The model under review builds one solid part; all positions refer to its coordinate system, in mm. Coordinates: 2 decimals unless noted, no trailing zeros. Order: outer loops, then holes, each group sorted by start corner. A loop starts at its lowest first (then second) coordinate and runs counter-clockwise, first axis right, second up. Notation, with made-up numbers: M 48.25,-39.75 L 99.25,-39.75 A29 ccw 99.25,-3.75 Z; hole C 67.25,22 d1. An arc over 180 degrees is marked long. Write each question's results on one line, items separated by ' | '.
from build123d import *

# Parameters (mm, degrees)
SKETCH1_W                                    = 40
SKETCH1_H                                    = 10
BOSS_EXTRUDE1_DEPTH                          = 3
CSK_FOR_M3_COUNTERSUNK_FLAT_HEAD_SCR_2_COUNT = 2
CSK_FOR_M3_COUNTERSUNK_FLAT_HEAD_SCR_2_PITCH = 28


with BuildPart() as part:
    # Sketch1 → Boss-Extrude1 (new body)
    with BuildSketch(Plane(origin=(0, 0, 0), x_dir=(1, 0, 0), z_dir=(0, 1, 0))):
        Rectangle(SKETCH1_W, SKETCH1_H)
    extrude(amount=BOSS_EXTRUDE1_DEPTH)

    # Sketch3 → CSK for M3 Countersunk Flat Head Screw1 (revolve, cut)
    with BuildSketch(Plane(origin=(-14, 3, 0), x_dir=(0, 0, 1), z_dir=(1, 0, 0))):
        Polygon((0, 0), (0, 3), (1.7, 3), (1.7, 1.45), (3.15, 0), align=None)
    csk_for_m3_countersunk_flat_head_screw1 = revolve(axis=Axis((-14, 9.35, 0), (0, -1, 0)), mode=Mode.SUBTRACT)

    # CSK for M3 Countersunk Flat Head Scr 2: CSK for M3 Countersunk Flat Head Screw1 ×2
    with Locations(*[(i * CSK_FOR_M3_COUNTERSUNK_FLAT_HEAD_SCR_2_PITCH, 0, 0) for i in range(1, CSK_FOR_M3_COUNTERSUNK_FLAT_HEAD_SCR_2_COUNT)]):
        add(csk_for_m3_countersunk_flat_head_screw1, mode=Mode.SUBTRACT)


solid = part.part
1) Take a section at B-B on z = 0. State the section outline as (x, y) points, plus the area to 3 significant figures.
Solutions:
outline: M -20,0 L -15.7,0 L -15.7,1.55 L -17.15,3 L -20,3 Z; M -12.3,0 L 12.3,0 L 12.3,1.55 L 10.85,3 L -10.85,3 L -12.3,1.55 Z; M 15.7,0 L 20,0 L 20,3 L 17.15,3 L 15.7,1.55 Z | area: 95.4 mm2
2) To check wall thickness, follow line 1 along X through (y, z) = (1.05, 0); line 2 along Z through (x, y) = (-14, 0.55); line 3 along X through (y, z) = (1.2, -1). State the ranges of each line that lie inside material, in increasing order.
Solutions:
line 1: -20 to -15.7, -12.3 to 12.3, 15.7 to 20 | line 2: -5 to -1.7, 1.7 to 5 | line 3: -20 to -15.37, -12.63 to 12.63, 15.37 to 20
3) Take a section at C-C on y = 1.15. State the section outline as (x, z) points.
Solutions:
outline: M -20,-5 L 20,-5 L 20,5 L -20,5 Z; hole C -14,0 d3.4; hole C 14,0 d3.4
4) For pin 1 (4 mm diameter, centred on x = 10, z = 3, fed in from -Y); pin 2 (2.5 mm diameter, centred on x = -14, z = 0, fed in from +Y), all flat-tipped, find the tip position at first contact; note any pin that passes through.
Solutions:
pin 1: y = 0 | pin 2: through
5) The part is to be moulded in two halves that separate along X. For faces 1 (the flat face through (-20, 1, 0)), 2 (the cylindrical face through (12.314, 0.786, -0.221)), 3 (the flat face through (0, 0, 0)), 4 (the flat face through (20, 1, 0)), say which applies: pulls with the +X half, pulls with the -X half, needs draft (parallel to the pull), parting line crosses it, or undercut.
Solutions:
face 1: pulls with the -X half | face 2: undercut | face 3: needs draft | face 4: pulls with the +X half
6) Take a section at A-A on x = -14. State the section outline as (y, z) points.
Solutions:
outline: M 0,-5 L 3,-5 L 3,-3.15 L 1.55,-1.7 L 0,-1.7 Z; M 0,1.7 L 1.55,1.7 L 3,3.15 L 3,5 L 0,5 Z
